```python
from build123d import *

# Parameters (mm, degrees)
F0_R     = 5
F1_DEPTH = 5


with BuildPart() as f1:
    # F0 (on Top) → F1 (new body)
    with BuildSketch(Plane.XY):
        with BuildLine():
            ThreePointArc((165.022992, 45.677721), (99.392758, 34.157347), (36.67612, 56.666677))
            ThreePointArc((36.67612, 56.666677), (-64.76451, 19.021258), (0.208612, -67.499678))
            ThreePointArc((0.208612, -67.499678), (-40.226954, -26.047967), (-29.270659, 30.813609))
            ThreePointArc((-29.270659, 30.813609), (-2.960146, 42.396787), (24.704722, 34.582173))
            ThreePointArc((24.704722, 34.582173), (98.597431, 9.139806), (175.511513, 22.984309))
            ThreePointArc((175.511513, 22.984309), (182.544206, 26.59511), (189.016125, 31.135037))
            ThreePointArc((189.016125, 31.135037), (194.510373, 42.034346), (184.288439, 48.704713))
            ThreePointArc((184.288439, 48.704713), (173.447839, 54.878805), (165.022992, 45.677721))
        make_face()
        with Locations((175, 45)):
            Circle(F0_R, mode=Mode.SUBTRACT)
    extrude(amount=F1_DEPTH)


solid = f1.part
```
Can you work these out from the model? Positions are in its coordinate system, mm. A direction names the side the tool comes from. Coordinates: 2 decimals unless noted, no trailing zeros. Loops run counter-clockwise (first coordinate to the right, second up) from the corner with the lowest first, then second, coordinate; pieces in that order, holes last. Notation, with made-up numbers: (-3, 76.5) -> (51, 76.5) arc R30 cw to (51, 112.5) -> close; hole circle Ø8 at (39.25, 59.25). An arc over 180 degrees is marked (long way). Put each result on its own line as item: value. Start each with the question number.
Q1. I want a section at A-A (z = 1.55). Write out the boundary of the cut face in (x, y), plus the area to 3 significant figures.
Q2. If I drill on line 1 (Y direction, x = 175, z = 2); line 2 (Y direction, x = 170.5, z = 4.4); line 3 (Y direction, x = 121.5, z = 3.1), over which ranges is the centre line in solid material (lowest first)? Write a range as [from, to].
Q3. I'm going to push flat-ended pins straight in: P1, Ø2, axis at x = -18.5, z = 3.5, coming from the -Y side; P2, Ø1, axis at y = -29, z = 3, coming from the +X side; P3, Ø3, axis at x = 124.5, z = 2.5, coming from the +Y side. Where does each tip first touch, or does it pass through?
Q4. I want a section at B-B (x = 133). Write out the boundary of the cut face in (y, z).
Q5. Thinking about a two-plate mould opening in X: for faces 1 (the face through (-64.247, 20.701, 2.465)), 2 (the face through (44, 30, 0)), 3 (the face through (97.49, 9.23, 2.46)), which applies, pulls with the +X half, pulls with the -X half, needs draft (parallel to the pull), parting line crosses it, or undercut?
Q6. I want a section at C-C (y = -35). Write out the boundary of the cut face in (x, z).
Q7. For faces 4 (the face through (100.33, 34.08, 2.46)), 5 (the face through (-3.37, 42.366, 2.465)), which set-ups out of +Z, -Z, +X, -X, +Y, -Y let a thin tool reach every point of the face, with its end or its side?
Taken from the geometry:
1. outline: (-29.27, 30.81) arc R42.5 cw to (24.7, 34.58) arc R155 ccw to (175.51, 22.98) arc R57.59 ccw to (189.02, 31.14) arc R9.15 ccw to (184.29, 48.7) arc R10 ccw to (165.02, 45.68) arc R130 cw to (36.68, 56.67) arc R67.5 ccw (long way) to (0.21, -67.5) arc R62.5 cw to start; hole circle Ø10 at (175, 45)
1. area: 8,560 mm2
2. line 1: y = [22.75, 40], [50, 55]
2. line 2: y = [20.77, 42.82], [47.18, 53.93]
2. line 3: y = [9.08, 34.15]
3. P1: stops at y = -65.19
3. P2: stops at x = -39.08
3. P3: stops at y = 34.61
4. outline: (10.33, 0) -> (35.65, 0) -> (35.65, 5) -> (10.33, 5) -> close
5. face 1: parting line crosses it
5. face 2: needs draft
5. face 3: undercut
6. outline: (-57.72, 0) -> (-36.77, 0) -> (-36.77, 5) -> (-57.72, 5) -> close
7. face 4: +Z, -Z, +Y
7. face 5: +Z, -Z
